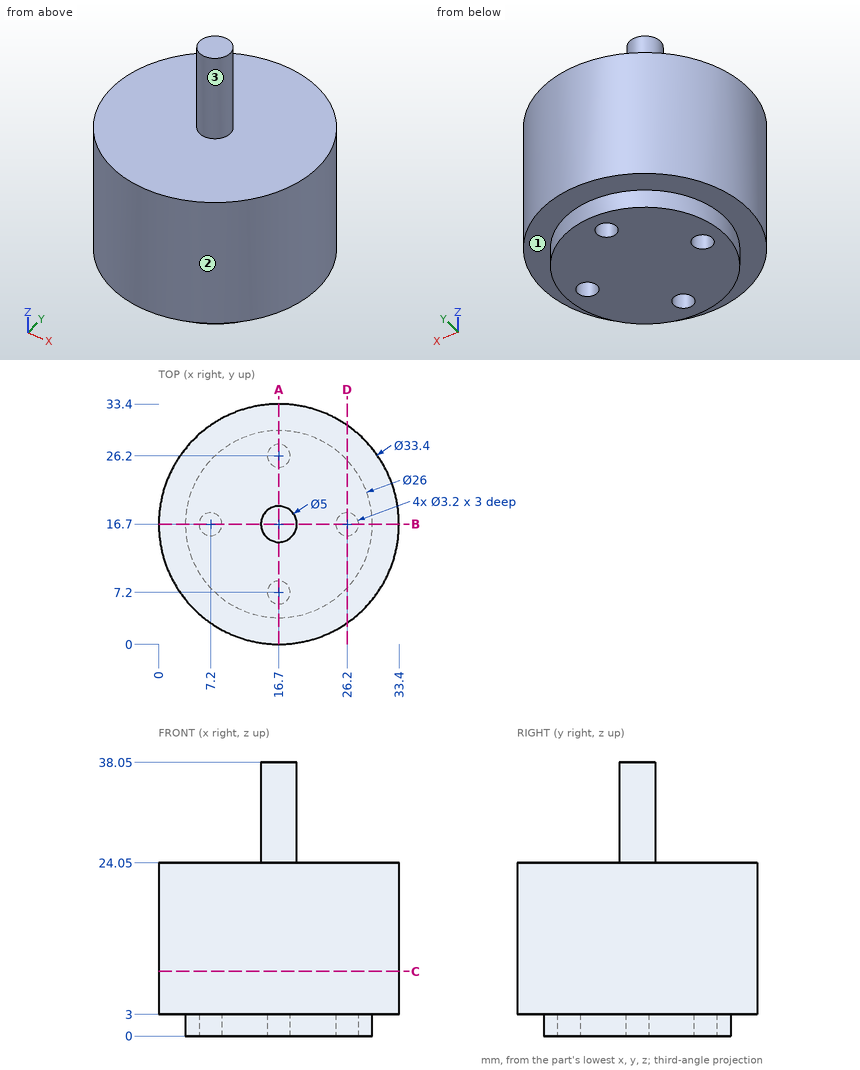
Geometry: see drawing. Coordinates: mm, zero at the bounding-box minimum. A direction names the side the tool comes from. Round coordinates to 2 decimals unless told otherwise and drop trailing zeros. Write each loop counter-clockwise with the first axis right and the second up, starting at its lowest first coordinate (ties: lowest second). Pieces come first, ordered by that corner, then holes. Notation, with made-up numbers: M 47,37.5 L 104,37.5 A23 cw 104,58.5 Z; hole C 81.5,27.5 d11. An arc over 180 degrees is marked long. Answer as a JSON object with one key per item and string values. Group by question number.
(1) Reachability of the marked faces 1, 2 and 3 from +Z, -Z, +X, -X, +Y, -Y: full face, straight path, thin tool, end or side. Return the list, or none.
(2) Section query A-A on x = 16.7. Output: boundary loops of the cut face in (y, z), then the cut area to 3 significant figures.
(3) Section query C-C on z = 9. Output: boundary loops of the cut face in (x, y), then the cut area to 3 significant figures.
(4) Ray query, line 1 (Y direction, x = 16.7, z = 1.75); line 2 (Z direction, x = 21.5, y = 30); line 3 (X direction, y = 7, z = 1). Return the intervals inside material, ascending. Write a range as [from, to].
(5) First-contact query: pin 1 (2.5 mm diameter, centred on x = 7.2, y = 16.7, fed in from -Z); pin 2 (6 mm diameter, centred on x = 11.5, z = 11, fed in from +Y); pin 3 (3 mm diameter, centred on x = 26.2, y = 16.7, fed in from +Z). Flat tips, straight axial feed; report the tip coordinate or a pass-through.
(6) Section query D-D on x = 26.2. Output: boundary loops of the cut face in (y, z), then the cut area to 3 significant figures.
Computed values:
{
 "1": {"face 1": "-Z", "face 2": "+Z, -Z", "face 3": "+Z"},
 "2": {"outline": "M 0,3 L 3.7,3 L 3.7,0 L 5.6,0 L 5.6,3 L 8.8,3 L 8.8,0 L 24.6,0 L 24.6,3 L 27.8,3 L 27.8,0 L 29.7,0 L 29.7,3 L 33.4,3 L 33.4,24.05 L 19.2,24.05 L 19.2,38.05 L 14.2,38.05 L 14.2,24.05 L 0,24.05 Z", "area": "832 mm^2"},
 "3": {"outline": "C 16.7,16.7 d33.4", "area": "876 mm^2"},
 "4": {"line 1": "[3.7, 5.6], [8.8, 24.6], [27.8, 29.7]", "line 2": "[3, 24.05]", "line 3": "[8.04, 15.11], [18.29, 25.36]"},
 "5": {"pin 1": "z = 3", "pin 2": "y = 33.25", "pin 3": "z = 24.05"},
 "6": {"outline": "M 2.97,3 L 7.83,3 L 7.83,0 L 15.1,0 L 15.1,3 L 18.3,3 L 18.3,0 L 25.57,0 L 25.57,3 L 30.43,3 L 30.43,24.05 L 2.97,24.05 Z", "area": "622 mm^2"}
}
